Geometry: see drawing. Coordinates: mm, zero at the bounding-box minimum. Give positions to 0.01 mm unless a question says otherwise; leave off trailing zeros. Order: outer loops, then holes, each group sorted by start corner. A loop starts at its lowest first (then second) coordinate and runs counter-clockwise, first axis right, second up. Notation, with made-up numbers: M 27,-14.75 L 44,-14.75 A31 ccw 44,19.25 Z; hole C 25,40.5 d11. An arc over 180 degrees is marked long. Answer as a JSON object with one key per item and string values. Group by question number.
1. Section query A-A (x = 9). Output: boundary loops of the cut face in (y, z).
2. Material intervals for L1, parallel to X at y = 12.75, z = 0.5 (1 decimal); L2, parallel to X at y = 14.75, z = 4; L3, parallel to Y at x = 12, z = 2.85 (1 decimal), sorted ascending. Write a range as [from, to].
3. Pull-direction query (X, two-part tool) for the marked faces 1, 2 and 3; classes: +X half, -X half, draft (parallel to the pull), parting line (faces both ways), or undercut.
4. Pin query (flat end, axial travel): P1, Ø1.4, axis at x = 5.5, y = 15.06, coming from the +Z side; P2, Ø1, axis at x = 2.5, z = 1, coming from the +Y side. Return the tip coordinate at first contact, or that it passes through.
5. Section query C-C (y = 12.25). Output: boundary loops of the cut face in (x, z) (1 decimal), plus the area to 3 significant figures.
6. Section query D-D (z = 1.9). Count the separate pieces of the cut face and the enclosed holes in it, plus the area to 3 significant figures.
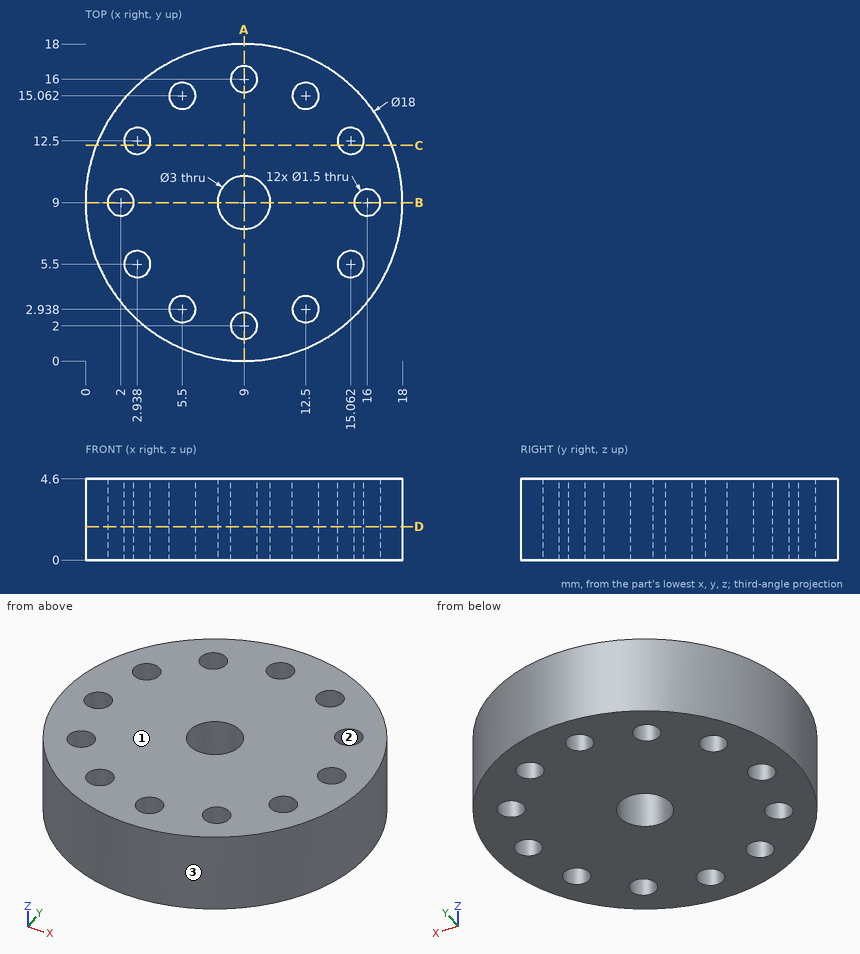
Answer sheet:
{
 "1": {"outline": "M 0,0 L 1.25,0 L 1.25,4.6 L 0,4.6 Z; M 2.75,0 L 7.5,0 L 7.5,4.6 L 2.75,4.6 Z; M 10.5,0 L 15.25,0 L 15.25,4.6 L 10.5,4.6 Z; M 16.75,0 L 18,0 L 18,4.6 L 16.75,4.6 Z"},
 "2": {"L1": "[0.8, 2.2], [3.6, 14.4], [15.8, 17.2]", "L2": "[2.08, 4.82], [6.18, 11.82], [13.18, 15.92]", "L3": "[0.5, 2.4], [3.5, 14.5], [15.6, 17.5]"},
 "3": {"face 1": "draft", "face 2": "undercut", "face 3": "parting line"},
 "4": {"P1": "through", "P2": "y = 15.71"},
 "5": {"outline": "M 0.6,0 L 2.2,0 L 2.2,4.6 L 0.6,4.6 Z; M 3.6,0 L 14.4,0 L 14.4,4.6 L 3.6,4.6 Z; M 15.8,0 L 17.4,0 L 17.4,4.6 L 15.8,4.6 Z", "area": "64.2 mm^2"},
 "6": {"separate pieces": "1", "enclosed holes": "13", "area": "226 mm^2"}
}
